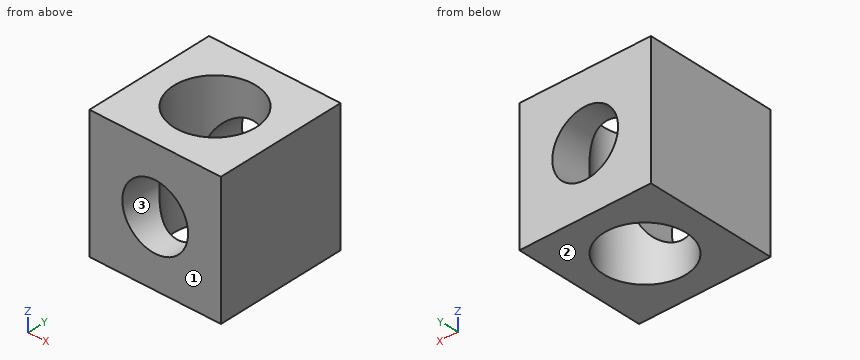
from build123d import *

# Parameters (mm, degrees)
SKETCH_W        = 40
SKETCH_H        = 40
PAD_DEPTH       = 40
SKETCH001_R     = 12.5
POCKET_DEPTH    = 40.001
SKETCH002_R     = 10
POCKET001_DEPTH = 40.001


with BuildPart() as part:
    # Sketch → Pad (new body)
    with BuildSketch(Plane.XY):
        Rectangle(SKETCH_W, SKETCH_H)
    extrude(amount=PAD_DEPTH)

    # Sketch001 (on Face6 of Pad) → Pocket (cut, through all)
    with BuildSketch(Plane.XY.offset(40)):
        Circle(SKETCH001_R)
    extrude(amount=-POCKET_DEPTH, mode=Mode.SUBTRACT)

    # Sketch002 (on Face6 of Pocket) → Pocket001 (cut, through all)
    with BuildSketch(Plane.XZ.offset(20)):
        with Locations((0, 20)):
            Circle(SKETCH002_R)
    extrude(amount=-POCKET001_DEPTH, mode=Mode.SUBTRACT)


solid = part.part
Geometry check sheet. Reference: the model listing, model coordinates, mm. Face numbers are marked on the shaded views. Coordinates: 2 decimals unless noted, no trailing zeros. Order: outer loops, then holes, each group sorted by start corner. A loop starts at its lowest first (then second) coordinate and runs counter-clockwise, first axis right, second up. Notation, with made-up numbers: (-25.75, 1) - (22.25, 1) arc R11 ccw to (22.25, 17) - close; hole circle Ø10 at (26.5, -9.75). An arc over 180 degrees is marked (long way). One line per item, written item: value.
(1) Sectioned sample at B-B (x = 0). Enter the section's corners in (y, z).
Data:
outline: (-20, 0) - (-12.5, 0) - (-12.5, 10) - (-20, 10) - close; (-20, 30) - (-12.5, 30) - (-12.5, 40) - (-20, 40) - close; (12.5, 0) - (20, 0) - (20, 10) - (12.5, 10) - close; (12.5, 30) - (20, 30) - (20, 40) - (12.5, 40) - close
(2) Thickness scan on probe 1 along X at (y, z) = (15, 20); probe 2 along Z at (x, y) = (0, 15); probe 3 along Y at (x, z) = (-10, 38.5). Record the ranges inside material, lowest first. Write a range as from..to.
Data:
probe 1: x = -20..-10, 10..20
probe 2: z = 0..10, 30..40
probe 3: y = -20..-7.5, 7.5..20
(3) Sectioned sample at D-D (x = -11.5). Enter the section's corners in (y, z), and give its area (3 significant figures).
Data:
outline: (-20, 0) - (-4.9, 0) - (-4.9, 40) - (-20, 40) - close; (4.9, 0) - (20, 0) - (20, 40) - (4.9, 40) - close
area: 1,210 mm^2
(4) Release check for a two-part mould opening along Z. For the marked faces 1, 2 and 3 record: +Z half, -Z half, draft (parallel to the pull), parting line (faces both ways), or undercut.
Data:
face 1: draft
face 2: -Z half
face 3: undercut
(5) Depth check by flat-ended pin: pin 1 Ø16 at (x, z) = (0, 20) entering from -Y. Enter the tip coordinate at first touch or a pass-through.
Data:
pin 1: passes through
(6) Sectioned sample at C-C (y = 0). Enter the section's corners in (x, z), and give its area (3 significant figures).
Data:
outline: (-20, 0) - (-12.5, 0) - (-12.5, 40) - (-20, 40) - close; (12.5, 0) - (20, 0) - (20, 40) - (12.5, 40) - close
area: 600 mm^2
(7) Sectioned sample at A-A (z = 20). Enter the section's corners in (x, y).
Data:
outline: (-20, -20) - (-10, -20) - (-10, -7.5) arc R12.5 cw to (-10, 7.5) - (-10, 20) - (-20, 20) - close; (10, -20) - (20, -20) - (20, 20) - (10, 20) - (10, 7.5) arc R12.5 cw to (10, -7.5) - close
